Model file for the job. Use its own axes, mm. Face numbers are marked on the shaded views. A direction names the side the tool comes from. Round coordinates to 2 decimals unless told otherwise and drop trailing zeros. Loops run counter-clockwise (first coordinate to the right, second up) from the corner with the lowest first, then second, coordinate; pieces in that order, holes last. Notation, with made-up numbers: M -16,-11.75 L 14,-11.75 A11 ccw 14,3.25 Z; hole C 13.25,-9 d10. An arc over 180 degrees is marked long. Use a Markdown table: item, result. Add a question column.
Item 1: Tool access for the marked faces 1 and 2: list every direction of +Z, -Z, +X, -X, +Y, -Y with a clear straight run to the whole face (end or side of a thin tool).
Item 2: Saw through at B-B on y = 0. Write the cut outline in (x, z), then the cut area to 3 significant figures.
Item 3: Saw through at A-A on z = 17.25. Write the cut outline in (x, y).
Item 4: Wall check: L1, parallel to Y at x = 0, z = 12.25; L2, parallel to Z at x = 3, y = 0.25; L3, parallel to Y at x = -2.5, z = 12. Give the ranges that are in metal, low to high. Write a range as from..to.
Item 5: Two-plate mould, pull along X, no slides. Class the marked faces 3, 4, 5 and 6: +X half, -X half, draft (parallel to the pull), parting line (faces both ways), or undercut.
Item 6: Pin check, flat tips, straight feed: P1, Ø2, axis at x = 2.5, z = 10, coming from the +Y side; P2, Ø1.3, axis at y = 2.5, z = 10, coming from the -X side; P3, Ø0.8, axis at y = -2, z = 15, coming from the -X side. Stop position of each tip, or through.
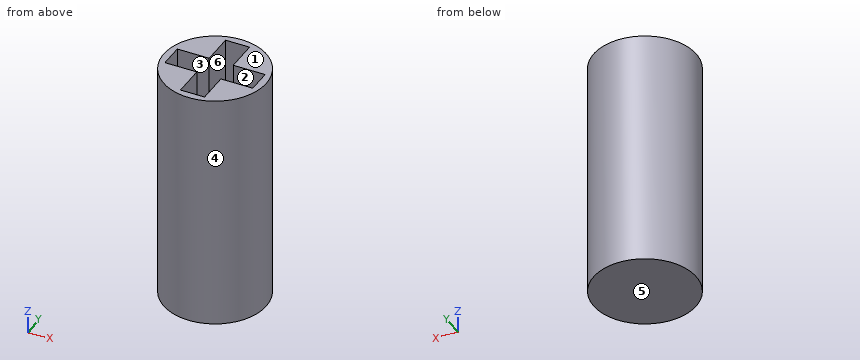
```python
from build123d import *

# Parameters (mm, degrees)
F0_R     = 4.25
F1_DEPTH = 20
F2_W     = 2.65
F2_H     = 2
F2_W_2   = 2
F2_H_2   = 2.65
F3_DEPTH = 19


with BuildPart() as f1:
    # F0 (on Top) → F1 (new body)
    with BuildSketch(Plane.XY):
        Circle(F0_R)
    extrude(amount=F1_DEPTH)

    # F2 (on face) → F3 (cut)
    with BuildSketch(Plane.XY.offset(20)):
        with Locations((2.325, 0)):
            Rectangle(F2_W, F2_H)
        with Locations((0, -2.325)):
            Rectangle(F2_W_2, F2_H_2)
        Rectangle(F2_W_2, F2_H)
        with Locations((-2.325, 0)):
            Rectangle(F2_W, F2_H)
        with Locations((0, 2.325)):
            Rectangle(F2_W_2, F2_H_2)
    extrude(amount=-F3_DEPTH, mode=Mode.SUBTRACT)


solid = f1.part
```
Entries:
| question | item | result |
|---|---|---|
| 1 | face 1 | +Z, +X, -X, +Y, -Y |
| 1 | face 2 | +Z |
| 2 | outline | M -4.25,0 L 4.25,0 L 4.25,20 L 3.65,20 L 3.65,1 L -3.65,1 L -3.65,20 L -4.25,20 Z |
| 2 | area | 31.3 mm2 |
| 3 | outline | C 0,0 d8.5; hole M -3.65,-1 L -1,-1 L -1,-3.65 L 1,-3.65 L 1,-1 L 3.65,-1 L 3.65,1 L 1,1 L 1,3.65 L -1,3.65 L -1,1 L -3.65,1 Z |
| 4 | L1 | -4.25..-3.65, 3.65..4.25 |
| 4 | L2 | 0..1 |
| 4 | L3 | -3.44..-1, 1..3.44 |
| 5 | face 3 | undercut |
| 5 | face 4 | parting line |
| 5 | face 5 | draft |
| 5 | face 6 | undercut |
| 6 | P1 | y = 3.98 |
| 6 | P2 | x = -3.83 |
| 6 | P3 | x = -3.94 |
